Work out the finished part from the listing and answer in its coordinate system (mm). A direction names the side the tool comes from. Give positions to 0.01 mm unless a question says otherwise; leave off trailing zeros. Order: outer loops, then holes, each group sorted by start corner. A loop starts at its lowest first (then second) coordinate and runs counter-clockwise, first axis right, second up.
```python
from build123d import *

# Parameters (mm, degrees)
SKETCH2_W                  = 349.5
SKETCH2_H                  = 196
SKETCH2_R                  = 3.06
SKETCH2_W_2                = 27
SKETCH2_H_2                = 62
BOSS_EXTRUDE1_DEPTH        = 50
M8X1_25_TAPPED_HOLE2_D     = 6.8
M8X1_25_TAPPED_HOLE2_DEPTH = 20
M8X1_25_TAPPED_HOLE2_TIP   = 2.042926105
M6X1_0_TAPPED_HOLE1_D      = 5
M6X1_0_TAPPED_HOLE1_DEPTH  = 20
M6X1_0_TAPPED_HOLE1_TIP    = 1.502151548
M6X1_0_TAPPED_HOLE2_D      = 5
M6X1_0_TAPPED_HOLE2_DEPTH  = 20
M6X1_0_TAPPED_HOLE2_TIP    = 1.502151548
M8X1_25_TAPPED_HOLE4_D     = 6.8
M8X1_25_TAPPED_HOLE4_DEPTH = 20
M8X1_25_TAPPED_HOLE4_TIP   = 2.042926105
M8X1_25_TAPPED_HOLE5_D     = 6.8
M8X1_25_TAPPED_HOLE5_DEPTH = 20
M8X1_25_TAPPED_HOLE5_TIP   = 2.042926105
HOLE1_D                    = 25
HOLE1_DEPTH                = 70
HOLE1_CBORE_D              = 29
HOLE1_CBORE_DEPTH          = 10


with BuildPart() as part:
    # Sketch2 → Boss-Extrude1 (new body)
    with BuildSketch(Plane.XY):
        with Locations((-34.75, 0)):
            Rectangle(SKETCH2_W, SKETCH2_H)
        with Locations((-29, -24)):
            Circle(SKETCH2_R, mode=Mode.SUBTRACT)
        with Locations((-29, -9)):
            Circle(SKETCH2_R, mode=Mode.SUBTRACT)
        with Locations((-58, 0)):
            Rectangle(SKETCH2_W_2, SKETCH2_H_2, mode=Mode.SUBTRACT)
        with BuildLine():
            Line((-5.06, 22), (-5.06, 5))
            ThreePointArc((-5.06, 5), (0, -0.06), (5.06, 5))
            Line((5.06, 5), (5.06, 22))
            ThreePointArc((5.06, 22), (0, 27.06), (-5.06, 22))
        make_face(mode=Mode.SUBTRACT)
    extrude(amount=BOSS_EXTRUDE1_DEPTH)

    # M8x1.25 Tapped Hole2
    with Locations(Plane(origin=(0, 0, 0), x_dir=(-0.9063077870366375, -0.4226182617407263, 0), z_dir=(0, 0, -1))):
        with Locations((74.606700972, 94.372083637), (120.24947324, -3.509157363), (-57.261082041, 32.881126554), (-11.618309773, -65.000114446)):
            Hole(M8X1_25_TAPPED_HOLE2_D / 2, depth=M8X1_25_TAPPED_HOLE2_DEPTH)
            with Locations((0, 0, -(M8X1_25_TAPPED_HOLE2_DEPTH + M8X1_25_TAPPED_HOLE2_TIP / 2))):  # 118° drill point
                Cone(0, M8X1_25_TAPPED_HOLE2_D / 2, M8X1_25_TAPPED_HOLE2_TIP, mode=Mode.SUBTRACT)

    # M6x1.0 Tapped Hole1
    with Locations(Plane(origin=(0, 0, 50), x_dir=(0.9063077870366375, 0.4226182617407263, 0), z_dir=(0, 0, 1))):
        with Locations((89.817329945, 53.007992242), (17.126988925, -102.876947128)):
            Hole(M6X1_0_TAPPED_HOLE1_D / 2, depth=M6X1_0_TAPPED_HOLE1_DEPTH)
            with Locations((0, 0, -(M6X1_0_TAPPED_HOLE1_DEPTH + M6X1_0_TAPPED_HOLE1_TIP / 2))):  # 118° drill point
                Cone(0, M6X1_0_TAPPED_HOLE1_D / 2, M6X1_0_TAPPED_HOLE1_TIP, mode=Mode.SUBTRACT)

    # M6x1.0 Tapped Hole2
    with Locations(Plane(origin=(0, 0, 50), x_dir=(0.9063077870366375, 0.4226182617407263, 0), z_dir=(0, 0, 1))):
        with Locations((-80.115380125, 132.248916319), (-152.805721144, -23.636023051)):
            Hole(M6X1_0_TAPPED_HOLE2_D / 2, depth=M6X1_0_TAPPED_HOLE2_DEPTH)
            with Locations((0, 0, -(M6X1_0_TAPPED_HOLE2_DEPTH + M6X1_0_TAPPED_HOLE2_TIP / 2))):  # 118° drill point
                Cone(0, M6X1_0_TAPPED_HOLE2_D / 2, M6X1_0_TAPPED_HOLE2_TIP, mode=Mode.SUBTRACT)

    # M8x1.25 Tapped Hole4
    with Locations(Plane(origin=(0, 0, 50), x_dir=(0.9063077870366375, 0.4226182617407263, 0), z_dir=(0, 0, 1))):
        with Locations((81.352699278, -128.41237604), (150.662094203, 20.222101034)):
            Hole(M8X1_25_TAPPED_HOLE4_D / 2, depth=M8X1_25_TAPPED_HOLE4_DEPTH)
            with Locations((0, 0, -(M8X1_25_TAPPED_HOLE4_DEPTH + M8X1_25_TAPPED_HOLE4_TIP / 2))):  # 118° drill point
                Cone(0, M8X1_25_TAPPED_HOLE4_D / 2, M8X1_25_TAPPED_HOLE4_TIP, mode=Mode.SUBTRACT)

    # M8x1.25 Tapped Hole5
    with Locations(Plane(origin=(0, 0, 50), x_dir=(0.9063077870366375, 0.4226182617407263, 0), z_dir=(0, 0, 1))):
        with Locations((-144.341090477, 157.784345231), (-213.650485402, 9.149868157)):
            Hole(M8X1_25_TAPPED_HOLE5_D / 2, depth=M8X1_25_TAPPED_HOLE5_DEPTH)
            with Locations((0, 0, -(M8X1_25_TAPPED_HOLE5_DEPTH + M8X1_25_TAPPED_HOLE5_TIP / 2))):  # 118° drill point
                Cone(0, M8X1_25_TAPPED_HOLE5_D / 2, M8X1_25_TAPPED_HOLE5_TIP, mode=Mode.SUBTRACT)

    # Hole1
    with Locations(Plane(origin=(83, -41, 50), x_dir=(1, 0, 0), z_dir=(0, 0, 1))):
        with Locations((0, 0), (0, 82), (-235.5, 82), (-235.5, 0)):
            CounterBoreHole(HOLE1_D / 2, HOLE1_CBORE_D / 2, HOLE1_CBORE_DEPTH, depth=HOLE1_DEPTH)


solid = part.part
```
1. The mould has two halves that part along Y. Classify faces 1 (the face through (-37, 1, 50)), 2 (the face through (72, -34, 40)): pulls with the +Y half, pulls with the -Y half, needs draft (parallel to the pull), parting line crosses it, or undercut.
Findings below:
face 1: needs draft
face 2: undercut
2. Which of the six approach directions +Z, -Z, +X, -X, +Y, -Y give full straight-line access (tool end or side, diameter ignored) to faces 3 (the face through (-146, 52, 40)), 4 (the face through (38.73, -57.32, 10.14)), 5 (the face through (-0.11, -0.06, 24.65))?
Findings below:
face 3: +Z
face 4: -Z
face 5: +Z, -Z
3. The part is cut by section D-D (x = -152.5). Write down the section's boundary in (y, z), then the cut area to 3 significant figures.
Findings below:
outline: (-98, 0) - (-53.5, 0) - (-53.5, 40) - (-55.5, 40) - (-55.5, 50) - (-98, 50) - close; (-28.5, 0) - (28.5, 0) - (28.5, 40) - (26.5, 40) - (26.5, 50) - (-26.5, 50) - (-26.5, 40) - (-28.5, 40) - close; (53.5, 0) - (98, 0) - (98, 50) - (55.5, 50) - (55.5, 40) - (53.5, 40) - close
area: 7,220 mm2
4. The part is cut by section C-C (z = 3.5). State how many separate pieces and enclosed holes the cut face has, then the cut area to 3 significant figures.
Findings below:
separate pieces: 1
enclosed holes: 12
area: 64,400 mm2
5. Straight lines are drawn through the part: probe 1 along X at (y, z) = (54, 6); probe 2 along Y at (x, z) = (83, 12.5); probe 3 along X at (y, z) = (-86, 39.25). For each, find the intervals that lie inside material, in ascending order.
Findings below:
probe 1: x = -209.5 to -110.9, -104.1 to 34.6, 41.4 to 140
probe 2: y = -98 to -53.5, -28.5 to 28.5, 53.5 to 98
probe 3: x = -209.5 to -131, -126 to 56.5, 61.5 to 140
6. The part is cut by section B-B (x = -52). Write down the section's boundary in (y, z), then the cut area to 3 significant figures.
Findings below:
outline: (-98, 0) - (-31, 0) - (-31, 50) - (-98, 50) - close; (31, 0) - (98, 0) - (98, 50) - (31, 50) - close
area: 6,700 mm2
7. The part is cut by section A-A (y = 10.5). Write down the section's boundary in (x, z).
Findings below:
outline: (-209.5, 0) - (-71.5, 0) - (-71.5, 50) - (-209.5, 50) - close; (-44.5, 0) - (-5.06, 0) - (-5.06, 50) - (-44.5, 50) - close; (5.06, 0) - (140, 0) - (140, 50) - (5.06, 50) - close
